```python
from build123d import *

# Parameters (mm, degrees)
SKETCH3_R           = 9.1313
CUT_EXTRUDE1_DEPTH  = 52.1843
SKETCH4_R           = 7.7343
CUT_EXTRUDE2_DEPTH  = 25.908
CHAMFER1_SIZE       = 3.9624
CHAMFER1_SIZE2      = 2.985882568
SKETCH5_R           = 11.56335
CUT_EXTRUDE3_DEPTH  = 20.19808
CUT_EXTRUDE3_TAPER  = 1.47
SKETCH6_R           = 12.081672541
CUT_EXTRUDE4_DEPTH  = 20.19808
SKETCH7_R           = 12.2174
BOSS_EXTRUDE1_DEPTH = 10.795


with BuildPart() as part:
    # Sweep1: sweep along a path in Sketch1
    with BuildLine(Plane.XY) as sweep1_path:
        Line((0, 0), (44.45, 0))
        Line((44.45, 0), (44.45, 25.908))
    # Sketch2 → Sweep1 (sweep)
    with BuildSketch(Plane(origin=(0, 0, 0), x_dir=(0, 0, -1), z_dir=(1, 0, 0))):
        Polygon((7.596312962, 13.1572), (-7.596312962, 13.1572), (-15.192625924, 0), (-7.596312962, -13.1572), (7.596312962, -13.1572), (15.192625924, 0), align=None)
    sweep(path=sweep1_path.line, transition=Transition.RIGHT)

    # Sketch3 → Cut-Extrude1 (cut)
    with BuildSketch(Plane.ZY):
        Circle(SKETCH3_R)
    extrude(amount=-CUT_EXTRUDE1_DEPTH, mode=Mode.SUBTRACT)

    # Sketch4 → Cut-Extrude2 (cut)
    with BuildSketch(Plane(origin=(0, 25.908, 0), x_dir=(1, 0, 0), z_dir=(0, 1, 0))):
        with Locations((44.45, 0)):
            Circle(SKETCH4_R)
    extrude(amount=-CUT_EXTRUDE2_DEPTH, mode=Mode.SUBTRACT)

    # Chamfer1
    chamfer1_edges = [part.edges().sort_by_distance(p)[0] for p in [
        (36.7157, 25.908, 0),
    ]]
    chamfer1_side = [part.faces().sort_by_distance(p)[0] for p in [
        (36.7157, 15.380996251, 0),
    ]]
    chamfer(chamfer1_edges, length=CHAMFER1_SIZE, length2=CHAMFER1_SIZE2, reference=chamfer1_side[0])

    # Sketch5 → Cut-Extrude3 (cut)
    with BuildSketch(Plane.ZY):
        Polygon((-7.596312962, 13.1572), (-15.192625924, 0), (-7.596312962, -13.1572), (7.596312962, -13.1572), (15.192625924, 0), (7.596312962, 13.1572), align=None)
        Circle(SKETCH5_R, mode=Mode.SUBTRACT)
    extrude(amount=-CUT_EXTRUDE3_DEPTH, taper=CUT_EXTRUDE3_TAPER, mode=Mode.SUBTRACT)

    # Sketch6 → Cut-Extrude4 (cut)
    with BuildSketch(Plane.ZY):
        Polygon((-15.192625924, 0), (-7.596312962, 13.1572), (7.596312962, 13.1572), (15.192625924, 0), (7.596312962, -13.1572), (-7.596312962, -13.1572), align=None)
        Circle(SKETCH6_R, mode=Mode.SUBTRACT)
    extrude(amount=-CUT_EXTRUDE4_DEPTH, mode=Mode.SUBTRACT)

    # Sketch7 → Boss-Extrude1 (add, symmetric)
    with BuildSketch(Plane(origin=(0, 25.908, 0), x_dir=(1, 0, 0), z_dir=(0, 1, 0))):
        Polygon((44.45, 18.330871047), (28.575, 9.165435523), (28.575, -9.165435523), (44.45, -18.330871047), (60.325, -9.165435523), (60.325, 9.165435523), align=None)
        with Locations((44.45, 0)):
            Circle(SKETCH7_R, mode=Mode.SUBTRACT)
    extrude(amount=BOSS_EXTRUDE1_DEPTH, both=True)


solid = part.part
```
Check sheet for the modelled part. Datum: model origin and axes. Units: mm. A direction names the side the tool comes from. Coordinates: 2 decimals unless noted, no trailing zeros. Loops run counter-clockwise (first coordinate to the right, second up) from the corner with the lowest first, then second, coordinate; pieces in that order, holes last. Notation, with made-up numbers: M -17,9.25 L 0,9.25 A24 ccw 0,25.25 Z; hole C 74.25,26.25 d1. An arc over 180 degrees is marked long. Answer as a JSON object with one key per item and string values.
1. Depth check by flat-ended pin: P1, Ø14.5, axis at y = 0, z = 0, coming from the -X side; P2, Ø2, axis at x = 8.5, y = 3.5, coming from the -Z side; P3, Ø12, axis at x = 45, z = -3.5, coming from the +Y side; P4, Ø3, axis at x = 13, z = 13.5, coming from the -Y side. Enter the tip coordinate at first touch or a pass-through.
Outcome:
{"P1": "x = 52.18", "P2": "z = -11.51", "P3": "y = 24.35", "P4": "through"}
2. Scan lines: L1, parallel to Z at x = 44.45, y = 13; L2, parallel to Z at x = 28.5, y = 0; L3, parallel to X at y = 15.5, z = 0 (3 decimals). Record each from-to range of solid material in increasing order. Write a range as from..to.
Outcome:
{"L1": "-15.19..-7.73, 7.73..15.19", "L2": "-15.19..-9.13, 9.13..15.19", "L3": "28.575..36.716, 52.184..60.325"}
3. Access from +Z, -Z, +X, -X, +Y, -Y to the whole of each face (thin tool, end or side, straight path). Record for faces 5 (the flat face through (57.607, 1, 0)), 6 (the flat face through (20.198, 6.9, -10.1)), 7 (the flat face through (31.293, 14, 0)), 8 (the cylindrical face through (38.75, 15.42, -5.23)), 9 (the flat face through (29.799, 5.025, -12.292)).
Outcome:
{"face 5": "+Z, -Z, +X, -Y", "face 6": "-X", "face 7": "+Z, -Z, -X", "face 8": "+Y", "face 9": "-Z, -X"}
4. Release check for a two-part mould opening along Y. For faces 1 (the flat face through (26, 13.157, 0)), 2 (the flat face through (43.2, 36.703, -12.31)), 3 (the flat face through (51.12, 4.32, -11.34)), 4 (the flat face through (35.01, -6.67, -11.34)) record: pulls with the +Y half, pulls with the -Y half, needs draft (parallel to the pull), parting line crosses it, or undercut.
Outcome:
{"face 1": "undercut", "face 2": "pulls with the +Y half", "face 3": "needs draft", "face 4": "pulls with the -Y half"}
5. Sectioned sample at A-A on y = 33. Record the cut outline in (x, z) (3 decimals), and give its area (3 significant figures).
Outcome:
{"outline": "M 28.575,-9.165 L 44.45,-18.331 L 60.325,-9.165 L 60.325,9.165 L 44.45,18.331 L 28.575,9.165 Z; hole C 44.45,0 d24.435", "area": "404 mm²"}
6. Sectioned sample at C-C on y = 17.5. Record the cut outline in (x, z) (3 decimals).
Outcome:
{"outline": "M 28.575,-9.165 L 44.45,-18.331 L 60.325,-9.165 L 60.325,9.165 L 44.45,18.331 L 28.575,9.165 Z; hole C 44.45,0 d15.469"}
7. Sectioned sample at B-B on z = -13.5. Record the cut outline in (x, y), and give its area (3 significant figures).
Outcome:
{"outline": "M 20.2,-2.93 L 47.38,-2.93 L 47.38,15.11 L 52.82,15.11 L 52.82,36.7 L 36.08,36.7 L 36.08,15.11 L 41.52,15.11 L 41.52,2.93 L 20.2,2.93 Z", "area": "592 mm²"}
